Geometry: final body of the model. Coordinates: model frame, mm. A direction names the side the tool comes from. Round coordinates to 2 decimals unless told otherwise and drop trailing zeros. Loops run counter-clockwise (first coordinate to the right, second up) from the corner with the lowest first, then second, coordinate; pieces in that order, holes last. Notation, with made-up numbers: (39.25, -29) - (75.25, -29) arc R9 ccw to (75.25, -17) - close; hole circle Ø3 at (4, 28.5). An arc over 180 degrees is marked (long way). Write item = value, one per line. Start each with the question number.
Item 1: Section B-B (z = -9). Return loops of the section in (x, y), plus the area to 3 significant figures.
Item 2: Section A-A (y = 8). Return loops of the section in (x, z).
Item 3: Section D-D (y = -0.5). Return loops of the section in (x, z), plus the area to 3 significant figures.
Item 4: Line query: line 1 (Y direction, x = 0, z = -14.15); line 2 (X direction, y = 12.3, z = 14.5); line 3 (X direction, y = 4, z = -4). Output: solid intervals per line, ascending. Write a range as from..to.
Item 5: Section C-C (x = -22.5). Return loops of the section in (y, z), plus the area to 3 significant figures.
Item 6: Access query for faces 1 (the flat face through (0, 4, 15)), 2 (the flat face through (19, 6, 14)), 3 (the flat face through (6, 11, 12)). Directions: +Z, -Z, +X, -X, +Y, -Y. A direction counts if a zero-diameter tool reaches every point of the face in a straight line with its end or side. Return the directions, or none.
Item 7: Draft query along X for faces 4 (the flat face through (-21, 11, 16)), 5 (the flat face through (-15, 9, 12)), 6 (the flat face through (5, -1, -14)). Return one class per face: pulls with the +X half, pulls with the -X half, needs draft (parallel to the pull), parting line crosses it, or undercut.
Item 8: First-contact query: pin 1 (2 mm diameter, centred on y = -0.5, z = 9.5, fed in from +X); pin 2 (9 mm diameter, centred on y = 9.5, z = -7, fed in from -X); pin 3 (5 mm diameter, centred on x = 0, z = 11, fed in from +Y); pin 4 (5 mm diameter, centred on x = 2.5, y = 9, fed in from -Z). Flat tips, straight axial feed; report the tip coordinate or a pass-through.
from build123d import *

# Parameters (mm, degrees)
SKETCH1_W           = 40
SKETCH1_H           = 30
BOSS_EXTRUDE1_DEPTH = 10
SKETCH5_W           = 40
SKETCH5_H           = 27
BOSS_EXTRUDE2_DEPTH = 3
SKETCH2_W           = 11
SKETCH2_H           = 24
CUT_EXTRUDE1_DEPTH  = 11
SKETCH4_W           = 6
SKETCH4_H           = 6
CUT_EXTRUDE2_DEPTH  = 8
SKETCH6_W           = 18
SKETCH6_H           = 16
CUT_EXTRUDE3_DEPTH  = 2
CHAMFER2_SIZE       = 3
BOSS_EXTRUDE3_DEPTH = 2
SKETCH9_R           = 1.5
CUT_EXTRUDE5_DEPTH  = 2
SKETCH11_W          = 40
SKETCH11_H          = 30
CUT_EXTRUDE6_DEPTH  = 1
CHAMFER3_SIZE       = 2
SKETCH14_W          = 6
SKETCH14_H          = 2
BOSS_EXTRUDE4_DEPTH = 4
SKETCH15_R          = 1.5
CUT_EXTRUDE7_DEPTH  = 4
CHAMFER7_SIZE       = 4
SKETCH16_W          = 13
SKETCH16_H          = 6.5
CUT_EXTRUDE8_DEPTH  = 3
SKETCH17_W          = 35
SKETCH17_H          = 24
CUT_EXTRUDE9_DEPTH  = 11


with BuildPart() as part:
    # Sketch1 → Boss-Extrude1 (new body)
    with BuildSketch(Plane(origin=(0, 0, 0), x_dir=(1, 0, 0), z_dir=(0, 1, 0))):
        Rectangle(SKETCH1_W, SKETCH1_H)
    extrude(amount=BOSS_EXTRUDE1_DEPTH)

    # Sketch5 → Boss-Extrude2 (add)
    with BuildSketch(Plane(origin=(0, 10, 0), x_dir=(1, 0, 0), z_dir=(0, 1, 0))):
        with Locations((0, -1.5)):
            Rectangle(SKETCH5_W, SKETCH5_H)
    extrude(amount=BOSS_EXTRUDE2_DEPTH)

    # Sketch2 → Cut-Extrude1 (cut)
    with BuildSketch(Plane(origin=(0, 13, 0), x_dir=(1, 0, 0), z_dir=(0, 1, 0))):
        with Locations((-12, 3)):
            Rectangle(SKETCH2_W, SKETCH2_H)
        with Locations((0, 3)):
            Rectangle(SKETCH2_W, SKETCH2_H)
        with Locations((12, 3)):
            Rectangle(SKETCH2_W, SKETCH2_H)
    extrude(amount=-CUT_EXTRUDE1_DEPTH, mode=Mode.SUBTRACT)

    # Sketch4 → Cut-Extrude2 (cut)
    with BuildSketch(Plane(origin=(0, 13, 0), x_dir=(1, 0, 0), z_dir=(0, 1, 0))):
        with Locations((-12, -12)):
            Rectangle(SKETCH4_W, SKETCH4_H)
        with Locations((0, -12)):
            Rectangle(SKETCH4_W, SKETCH4_H)
        with Locations((12, -12)):
            Rectangle(SKETCH4_W, SKETCH4_H)
    extrude(amount=-CUT_EXTRUDE2_DEPTH, mode=Mode.SUBTRACT)

    # Sketch6 → Cut-Extrude3 (cut)
    with BuildSketch(Plane(origin=(0, 13, 0), x_dir=(1, 0, 0), z_dir=(0, 1, 0))):
        with Locations((0, -7)):
            Rectangle(SKETCH6_W, SKETCH6_H)
    extrude(amount=-CUT_EXTRUDE3_DEPTH, mode=Mode.SUBTRACT)

    # Chamfer2
    chamfer2_edges = [part.edges().sort_by_distance(p)[0] for p in [
        (18.75, 10, -12),
        (6, 10, -12),
        (-6, 10, -12),
        (-18.75, 10, -12),
    ]]
    chamfer(chamfer2_edges, length=CHAMFER2_SIZE - 0.0001)  # a hair under: the kernel refuses the full size

    # Sketch8 → Boss-Extrude3 (add)
    with BuildSketch(Plane(origin=(0, 13, 0), x_dir=(1, 0, 0), z_dir=(0, 1, 0))):
        Polygon((20, -10), (27.39103626, -13.061467459), (24.712252234, -19.528624186), (15, -15.50567759), (15, -15), (17.5, -9), align=None)
    boss_extrude3 = extrude(amount=-BOSS_EXTRUDE3_DEPTH)

    # Mirror1: Boss-Extrude3 across plane
    add(boss_extrude3.mirror(Plane(origin=(0, 0, 0), x_dir=(0, 0, 1), z_dir=(1, 0, 0))))

    # Sketch9 → Cut-Extrude5 (cut)
    with BuildSketch(Plane.XZ.offset(-11)):
        with Locations(Location((-22.5, 14.5, 0), (0, 0, 270))):
            Circle(SKETCH9_R)
        with Locations(Location((22.5, 14.5, 0), (0, 0, 270))):
            Circle(SKETCH9_R)
    extrude(amount=-CUT_EXTRUDE5_DEPTH, mode=Mode.SUBTRACT)

    # Sketch11 → Cut-Extrude6 (cut)
    with BuildSketch(Plane.XZ):
        Rectangle(SKETCH11_W, SKETCH11_H)
    extrude(amount=-CUT_EXTRUDE6_DEPTH, mode=Mode.SUBTRACT)

    # Chamfer3
    chamfer3_edges = [part.edges().sort_by_distance(p)[0] for p in [
        (20, 6, 15),
        (-20, 6, 15),
        (0, 1, 15),
    ]]
    chamfer(chamfer3_edges, length=CHAMFER3_SIZE)

    # Sketch14 → Boss-Extrude4 (add)
    with BuildSketch(Plane.XZ.offset(-1)):
        with Locations((0, -14)):
            Rectangle(SKETCH14_W, SKETCH14_H)
    extrude(amount=BOSS_EXTRUDE4_DEPTH)

    # Sketch15 → Cut-Extrude7 (cut)
    with BuildSketch(Plane(origin=(0, 0, -15), x_dir=(-1, 0, 0), z_dir=(0, 0, -1))):
        with Locations((0, -0.5)):
            Circle(SKETCH15_R)
    extrude(amount=-CUT_EXTRUDE7_DEPTH, mode=Mode.SUBTRACT)

    # Chamfer7
    chamfer7_edges = [part.edges().sort_by_distance(p)[0] for p in [
        (3, 1, -14),
        (-3, 1, -14),
    ]]
    chamfer(chamfer7_edges, length=CHAMFER7_SIZE - 0.0001)  # a hair under: the kernel refuses the full size

    # Sketch16 → Cut-Extrude8 (cut)
    with BuildSketch(Plane(origin=(0, 13, 0), x_dir=(1, 0, 0), z_dir=(0, 1, 0))):
        with Locations((0, 11.75)):
            Rectangle(SKETCH16_W, SKETCH16_H)
    extrude(amount=-CUT_EXTRUDE8_DEPTH, mode=Mode.SUBTRACT)

    # Sketch17 → Cut-Extrude9 (cut)
    with BuildSketch(Plane(origin=(0, 13, 0), x_dir=(1, 0, 0), z_dir=(0, 1, 0))):
        with Locations((0, 3)):
            Rectangle(SKETCH17_W, SKETCH17_H)
    extrude(amount=-CUT_EXTRUDE9_DEPTH, mode=Mode.SUBTRACT)


solid = part.part
Taken from the geometry:
q1.outline = (-20, 1) - (20, 1) - (20, 13) - (17.5, 13) - (17.5, 2) - (-17.5, 2) - (-17.5, 13) - (-20, 13) - close
q1.area = 95.0 mm^2
q2.outline = (-20, -15) - (-17.5, -15) - (-17.5, 9) - (-15, 9) - (-15, 15) - (-18, 15) - (-20, 13) - close; (-9, 9) - (-3, 9) - (-3, 15) - (-9, 15) - close; (3, 9) - (9, 9) - (9, 15) - (3, 15) - close; (15, 9) - (17.5, 9) - (17.5, -15) - (20, -15) - (20, 13) - (18, 15) - (15, 15) - close
q3.outline = (-5.5, -15) - (-1.5, -15) - (-1.5, -13) - (-5.5, -13) - close; (1.5, -15) - (5.5, -15) - (5.5, -13) - (1.5, -13) - close
q3.area = 16.0 mm^2
q4.line_1 = -3..-2, 1..2
q4.line_2 = -26.8..-24, -21..-15, 15..21, 24..26.8
q4.line_3 = -20..-17.5, 17.5..20
q5.outline = (11, 11.04) - (13, 11.04) - (13, 13) - (11, 13) - close; (11, 16) - (13, 16) - (13, 18.61) - (11, 18.61) - close
q5.area = 9.15 mm^2
q6.face_1 = +Z, +X, -X, -Y
q6.face_2 = +Z, +X, -Y
q6.face_3 = +Z, -Z, +Y
q7.face_4 = needs draft
q7.face_5 = undercut
q7.face_6 = pulls with the +X half
q8.pin_1 = through
q8.pin_2 = -20
q8.pin_3 = 5
q8.pin_4 = 9
